```python
from build123d import *

# Parameters (mm, degrees)
F1_DEPTH  = 9
F2_R      = 10.5
F3_DEPTH  = 3
F4_R      = 5
F5_DEPTH  = 95
F7_D      = 3.2
F7_DEPTH  = 5
F7_TIP    = 0.9613769904
F9_D      = 4.1
F9_DEPTH  = 18.5
F9_TIP    = 1.231764269
F11_D     = 4.1
F11_DEPTH = 100
F11_TIP   = 1.231764269
F13_D     = 5.5
F13_DEPTH = 9
F13_TIP   = 1.6523667023


with BuildPart() as f1:
    # F0 (on Top) → F1 (new body)
    with BuildSketch(Plane.XY):
        with BuildLine():
            Line((-17.435, 15), (-17.4355957742, 15))
            ThreePointArc((-17.4355957742, 15), (-23, 0), (-17.4355957742, -15))
            Line((-17.4355957742, -15), (-17.435, -15))
            Line((-17.435, -15), (17.435, -15))
            Line((17.435, -15), (17.4355957742, -15))
            ThreePointArc((17.4355957742, -15), (23, 0), (17.4355957742, 15))
            Line((17.4355957742, 15), (17.435, 15))
            Line((17.435, 15), (-17.435, 15))
        make_face()
    extrude(amount=F1_DEPTH)

    # F2 (on face) → F3 (join)
    with BuildSketch(Plane(origin=(0, 0, 0), x_dir=(1, 0, 0), z_dir=(0, 0, -1))):
        Circle(F2_R)
    extrude(amount=F3_DEPTH)

    # F4 (on face) → F5 (join)
    with BuildSketch(Plane.XY.offset(9)):
        Circle(F4_R)
    extrude(amount=F5_DEPTH)

    # F7 (one way)
    with BuildSketch(Plane(origin=(0, 0, 0), x_dir=(1, 0, 0), z_dir=(0, 1, 0))):
        with Locations((0, -31)):
            Circle(F7_D / 2)
    extrude(amount=-F7_DEPTH, mode=Mode.SUBTRACT)
    with Locations(Plane(origin=(0, 0, 0), x_dir=(1, 0, 0), z_dir=(0, 1, 0))):
        with Locations((0, -31)):
            with Locations((0, 0, -(F7_DEPTH + F7_TIP / 2))):  # 118° drill point
                Cone(0, F7_D / 2, F7_TIP, mode=Mode.SUBTRACT)

    # F9
    with Locations(Plane.XZ.offset(15)):
        with Locations((0, 4)):
            Hole(F9_D / 2, depth=F9_DEPTH)
            with Locations((0, 0, -(F9_DEPTH + F9_TIP / 2))):  # 118° drill point
                Cone(0, F9_D / 2, F9_TIP, mode=Mode.SUBTRACT)

    # F11
    with Locations(Plane.XY.offset(104)):
        with Locations((0, 0)):
            Hole(F11_D / 2, depth=F11_DEPTH)
            with Locations((0, 0, -(F11_DEPTH + F11_TIP / 2))):  # 118° drill point
                Cone(0, F11_D / 2, F11_TIP, mode=Mode.SUBTRACT)

    # F13
    with Locations(Plane.XY.offset(9)):
        with Locations((-16, 9), (16, -9)):
            Hole(F13_D / 2, depth=F13_DEPTH)
            with Locations((0, 0, -(F13_DEPTH + F13_TIP / 2))):  # 118° drill point
                Cone(0, F13_D / 2, F13_TIP, mode=Mode.SUBTRACT)


solid = f1.part
```
Geometry check sheet. Reference: the model listing, model coordinates, mm. A direction names the side the tool comes from. Round coordinates to 2 decimals unless told otherwise and drop trailing zeros. Order: outer loops, then holes, each group sorted by start corner. A loop starts at its lowest first (then second) coordinate and runs counter-clockwise, first axis right, second up. Notation, with made-up numbers: M 77,57.25 L 92,57.25 A15 cw 92,68.25 Z; hole C -22.5,-32 d4. An arc over 180 degrees is marked long. Write item = value, one per line.
Q1. Release check for a two-part mould opening along Y. For faces 5 (the cylindrical face through (23, 0, 4)), 6 (the cylindrical face through (0.267, 2.033, 53.3)), 7 (the cylindrical face through (-13.253, 9.121, 4.437)), 8 (the flat face through (-5.4, 0.2, 9)) record: released by +Y, released by -Y, zero draft, split by the parting line, or undercut.
Answer block:
face_5 = split by the parting line
face_6 = undercut
face_7 = undercut
face_8 = zero draft
Q2. Section check B-B (y = -9). Enter the section's corners in (x, z), plus the area to 3 significant figures.
Answer block:
outline = M -21.17,0 L -5.41,0 L -5.41,-3 L 5.41,-3 L 5.41,0 L 13.25,0 L 13.25,9 L -21.17,9 Z; M 18.75,0 L 21.17,0 L 21.17,9 L 18.75,9 Z; hole C 0,4 d4.1
area = 351 mm^2
Q3. Section check D-D (y = 9). Enter the section's corners in (x, z), plus the area to 3 significant figures.
Answer block:
outline = M -21.17,0 L -18.75,0 L -18.75,9 L -21.17,9 Z; M -13.25,0 L -5.41,0 L -5.41,-3 L 5.41,-3 L 5.41,0 L 21.17,0 L 21.17,9 L -13.25,9 Z
area = 364 mm^2
Q4. Section check A-A (x = 16). Enter the section's corners in (y, z).
Answer block:
outline = M -15,0 L -11.75,0 L -11.75,9 L -15,9 Z; M -6.25,0 L 15,0 L 15,9 L -6.25,9 Z
Q5. Section check C-C (z = 17.5). Enter the section's corners in (x, y), plus the area to 3 significant figures.
Answer block:
outline = C 0,0 d10; hole C 0,0 d4.1
area = 65.3 mm^2
Q6. Set-up check for faces 1 (the flat face through (-11, 0, 0)), 2 (the cylindrical face through (-1.08, -4.88, 55.84)), 3 (the cylindrical face through (0.444, -5.62, 1.999)), 4 (the cylindrical face through (-23, 0, 4)): record each of +Z, -Z, +X, -X, +Y, -Y from which the full face is reachable in a straight line by a thin tool's end or side.
Answer block:
face_1 = -Z
face_2 = +Z
face_3 = -Y
face_4 = +Z, -Z, -X
Q7. Scan lines: line 1 (Z direction, x = 0, y = -5.75); line 2 (Y direction, x = -16, z = 6); line 3 (X direction, y = -9, z = 2.5). Record each from-to range of solid material in increasing order.
Answer block:
line_1 = -3 to 1.95, 6.05 to 9
line_2 = -15 to 6.25, 11.75 to 15
line_3 = -21.17 to -1.4, 1.4 to 13.25, 18.75 to 21.17
Q8. Depth check by flat-ended pin: pin 1 Ø5 at (y, z) = (4.5, 36.5) entering from -X; pin 2 Ø8 at (x, z) = (-0.5, 36) entering from +Y; pin 3 Ø10 at (y, z) = (-9.5, 50.5) entering from +X; pin 4 Ø4.5 at (x, y) = (16, -9) entering from +Z. Enter the tip coordinate at first touch or a pass-through.
Answer block:
pin_1 = -4.58
pin_2 = 5
pin_3 = 2.18
pin_4 = through
